Print and shaded views of the part. All mm, measured from the part's lowest x, y and z. Coordinates: 2 decimals unless noted, no trailing zeros. Loops run counter-clockwise (first coordinate to the right, second up) from the corner with the lowest first, then second, coordinate; pieces in that order, holes last. Notation, with made-up numbers: M 80.5,-19 L 113.5,-19 A11 cw 113.5,-10 Z; hole C 33.5,-39.5 d1. An arc over 180 degrees is marked long. One line per question, with ' | ' between items. Start each with the question number.
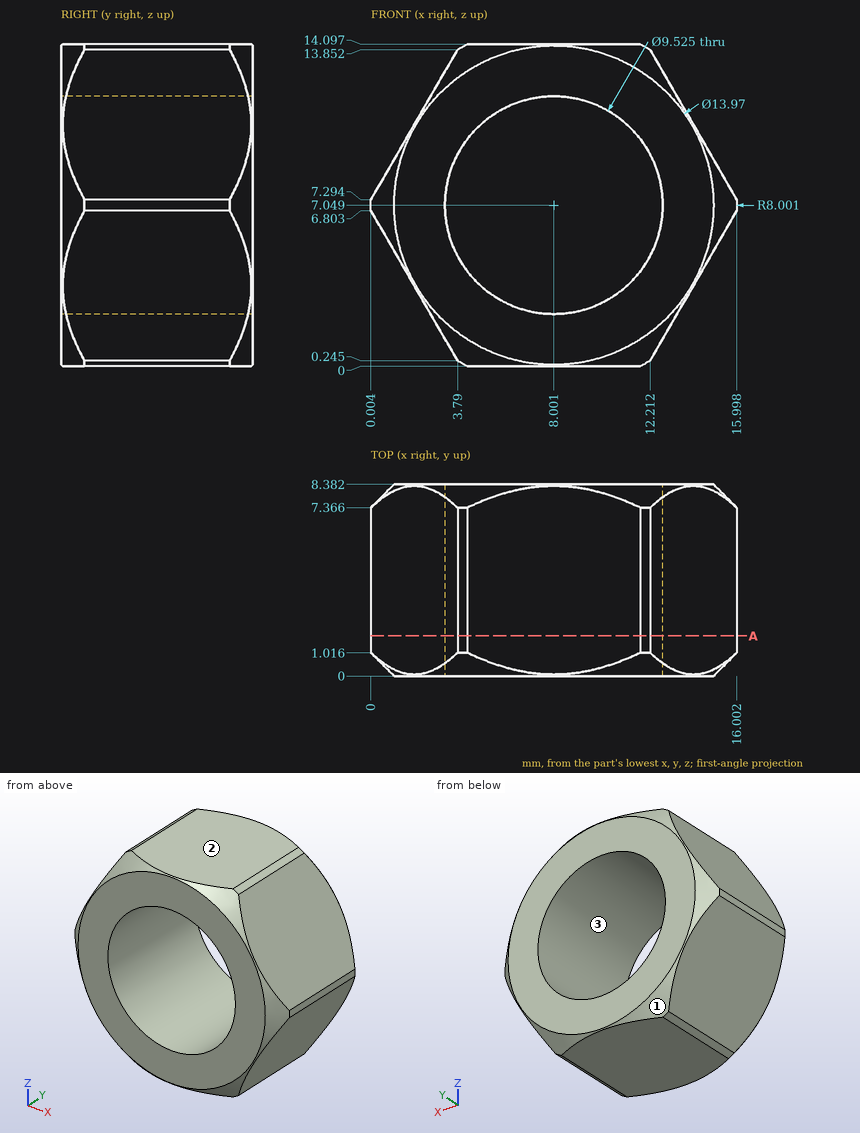
(1) Drill centre lines: line 1 (X direction, y = 1.75, z = 7); line 2 (Z direction, x = 6.5, y = 5); line 3 (Z direction, x = 6.25, y = 6.5). Where is each one in solid material? Low to high. Write a range as [from, to].
(2) Two-plate mould, pull along Z, no slides. Class the marked faces 1, 2 and 3: pulls with the +Z half, pulls with the -Z half, needs draft (parallel to the pull), parting line crosses it, or undercut.
(3) Band-saw the part on A-A on y = 1.75. Write the cut outline in (x, z) (1 decimal), then the cut area to 3 significant figures.
Computed values:
1) line 1: [0, 3.24], [12.76, 16] | line 2: [0, 2.53], [11.57, 14.1] | line 3: [0, 2.62], [11.48, 14.1]
2) face 1: parting line crosses it | face 2: pulls with the +Z half | face 3: undercut
3) outline: M 0,6.8 L 3.8,0.2 A8 ccw 4.2,0 L 11.8,0 A8 ccw 12.2,0.2 L 16,6.8 A8 ccw 16,7.3 L 12.2,13.9 A8 ccw 11.8,14.1 L 4.2,14.1 A8 ccw 3.8,13.9 L 0,7.3 A8 ccw Z; hole C 8,7 d9.5 | area: 101 mm^2
